from build123d import *

# Parameters (mm, degrees)
SKETCH001_R        = 5.72703
POCKET_DEPTH       = 113.912459
POLARPATTERN_COUNT = 4
SKETCH002_R        = 7
POCKET001_DEPTH    = 23


with BuildPart() as part:
    # Sketch → Revolution (revolve)
    with BuildSketch(Plane.XY):
        with BuildLine():
            ThreePointArc((4.191612, 0), (3.089028, 4.826759), (0, 8.696022))
            Line((0, 8.696022), (0, 12.478185))
            Line((0, 12.478185), (-3.839461, 12.478185))
            ThreePointArc((-8.326538, 9.189423), (-6.01736, 10.744248), (-3.839461, 12.478185))
            Line((-8.326538, 9.189423), (-17.102989, 9.162301))
            Line((-17.102989, 9.162301), (-17.277503, 8.538994))
            Line((-17.277503, 8.538994), (-21.978689, 8.538994))
            Line((-21.978689, 8.538994), (-22.338589, 9.1623))
            Line((-22.338589, 9.1623), (-23.808388, 9))
            Line((-23.808388, 9), (-23.808388, 0))
            Line((-23.808388, 0), (4.191612, 0))
        make_face()
    revolve(axis=Axis((0, 0, 0), (1, 0, 0)))

    # Sketch001 (on Face2 of Revolution) → Pocket (cut, through all)
    with BuildSketch(Plane.YZ):
        with Locations((14.923323, 0)):
            Circle(SKETCH001_R)
    pocket = extrude(amount=-POCKET_DEPTH, mode=Mode.SUBTRACT)

    # PolarPattern: Pocket ×4 about axis
    polarpattern_axis = Axis((0, 0, 0), (1, 0, 0))
    for i in range(1, POLARPATTERN_COUNT):
        add(pocket.rotate(polarpattern_axis, i * 360 / POLARPATTERN_COUNT), mode=Mode.SUBTRACT)

    # Sketch002 (on Face17 of PolarPattern) → Pocket001 (cut)
    with BuildSketch(Plane(origin=(-23.808388, 0, 0), x_dir=(0, -1, 0), z_dir=(-1, 0, 0))):
        Circle(SKETCH002_R)
    extrude(amount=-POCKET001_DEPTH, mode=Mode.SUBTRACT)


solid = part.part
Verification items for the finished model (mm, model axes). A direction names the side the tool comes from. Give positions to 0.01 mm unless a question says otherwise; leave off trailing zeros. Loops run counter-clockwise (first coordinate to the right, second up) from the corner with the lowest first, then second, coordinate; pieces in that order, holes last.
1) Thickness scan on line 1 along Z through (x, y) = (-16, 0); line 2 along Y through (x, z) = (-20.5, -3.75); line 3 along Y through (x, z) = (-22.25, 1.25). Record the ranges inside material, lowest first.
2) Sectioned sample at A-A, the plane x = -6. Enter the section's corners in (y, z).
3) Depth check by flat-ended pin: pin 1 Ø12 at (y, z) = (-4, -7.5) entering from +X; pin 2 Ø6 at (y, z) = (0, 8.5) entering from +X; pin 3 Ø5 at (x, z) = (-5.5, 1.5) entering from -Y. Enter the tip coordinate at first touch or a pass-through.
4) Sectioned sample at B-B, the plane x = -11.25. Enter the section's corners in (y, z), then the cut area to 3 significant figures.
5) Set-up check for faces 4 (the cylindrical face through (-1.947, -8.773, 8.873)), 5 (the conical face through (-12.78, 8.75, 2.76)): record each of +Z, -Z, +X, -X, +Y, -Y from which the full face is reachable in a straight line by a thin tool's end or side.
6) Draft check along Y on faces 1 (the flat face through (0, 2, -9)), 2 (the cylindrical face through (-19.66, -8.53, 0.38)), 3 (the flat face through (-0.808, 0, 0)). Enter one of: pulls with the +Y half, pulls with the -Y half, needs draft (parallel to the pull), parting line crosses it, or undercut.
Answers:
1. line 1: z = -9.17 to -7, 7 to 9.17
1. line 2: y = -7.67 to -5.91, 5.91 to 7.67
1. line 3: y = -8.92 to -6.89, 6.89 to 8.92
2. outline: (-10.24, -3.3) arc R10.76 ccw to (-3.3, -10.24) arc R5.73 cw to (3.3, -10.24) arc R10.76 ccw to (10.24, -3.3) arc R5.73 cw to (10.24, 3.3) arc R10.76 ccw to (3.3, 10.24) arc R5.73 cw to (-3.3, 10.24) arc R10.76 ccw to (-10.24, 3.3) arc R5.73 cw to start; hole circle Ø14 at (0, 0)
3. pin 1: stops at x = 3.91
3. pin 2: stops at x = 2.74
3. pin 3: stops at y = -10.78
4. outline: circle Ø18.36 at (0, 0); hole circle Ø14 at (0, 0)
4. area: 111 mm2
5. face 4: +Z, +X, -X, -Y
5. face 5: -X
6. face 1: needs draft
6. face 2: parting line crosses it
6. face 3: undercut
